Could you check a few things on this model? Use its own coordinates, in mm. A direction names the side the tool comes from. Coordinates: 2 decimals unless noted, no trailing zeros. Order: outer loops, then holes, each group sorted by start corner. A loop starts at its lowest first (then second) coordinate and runs counter-clockwise, first axis right, second up. Notation, with made-up numbers: (47.5, 57.25) - (86.5, 57.25) arc R26 cw to (86.5, 92.25) - close; hole circle Ø4 at (52, 25). An arc over 180 degrees is marked (long way). Answer as CSV lines item,"result". Start each with the question number.
1. I want a section at C-C, the plane z = 0.75. List the corners of the cut face in (x, y) for me, and give its area (3 significant figures).
2. For faces 1 (the face through (0, 2, 2)), 2 (the face through (-5, 0, 2)), which set-ups out of +Z, -Z, +X, -X, +Y, -Y let a thin tool reach every point of the face, with its end or its side?
3. I want a section at B-B, the plane x = 0. List the corners of the cut face in (y, z) for me, and give its area (3 significant figures).
4. I need wall thicknesses on probe 1 along Y at (x, z) = (-2, 0.6); probe 2 along X at (y, z) = (0.9, 1.55). Which ranges of each line are inside material? Lowest first, please.
5. I want a section at A-A, the plane y = -1.55. List the corners of the cut face in (x, z) for me.
6. Thinking about a two-plate mould opening in Y: for faces 3 (the face through (-4, 0, 2)), 4 (the face through (0, 3, 2)), 5 (the face through (0, -3, 2)), which applies, released by +Y, released by -Y, zero draft, split by the parting line, or undercut?
Autodesk Inventor part; units mm, degrees
ref_plane "Work Plane1" through (0, 0, 2) normal (0, 0, 1) x (1, 0, 0)
ref_plane "YZ Plane" through (0, 0, 0) normal (1, 0, 0) x (0, 1, 0)
ref_plane "XZ Plane" through (0, 0, 0) normal (0, 1, 0) x (-1, 0, 0)
sketch "Sketch1" plane through (0, 0, 0) normal (0, 0, 1) x (1, 0, 0)
  line L0 (-4, 2) -> (4, 2)
  line L1 (4, 2) -> (4, -2)
  line L2 (4, -2) -> (-4, -2)
  line L3 (-4, -2) -> (-4, 2)
  line L4 (5, 3) -> (-5, 3)
  line L5 (-5, 3) -> (-5, -3)
  line L6 (-5, -3) -> (5, -3)
  line L7 (5, -3) -> (5, 3)
  point P0 (0, 0)
  dimension "d0" = 8
  dimension "d1" = 4
  dimension "d2" = 2
  dimension "d3" = 4
  dimension "d5" = 1
extrude "Extrusion1" add sketch "Sketch1" along normal blind 4
ref_plane "Work Plane1" through (0, 0, 2) normal (0, 0, 1) x (1, 0, 0)
sketch "Sketch2" plane through (0, 0, 2) normal (0, 0, 1) x (1, 0, 0)
  line L0 (0, 0) -> (5.4411, 0) construction
  point P0 (2.25, 1)
  point P1 (0.75, 1)
  point P2 (-0.75, 1)
  point P3 (-2.25, 1)
  dimension "d11" = 1.5
  dimension "d16" = 2.25
  dimension "d17" = 1
properties part number "CrimpSocket"
Solved:
1,outline,"(-5, -3) - (5, -3) - (5, 3) - (-5, 3) - close; hole (-4, -2) - (4, -2) - (4, 2) - (-4, 2) - close"
1,area,"28.0 mm2"
2,face 1,"+Z, -Z"
2,face 2,"+Z, -Z, -X, +Y, -Y"
3,outline,"(-3, 0) - (-2, 0) - (-2, 4) - (-3, 4) - close; (2, 0) - (3, 0) - (3, 4) - (2, 4) - close"
3,area,"8.00 mm2"
4,probe 1,"y = -3 to -2, 2 to 3"
4,probe 2,"x = -5 to -4, 4 to 5"
5,outline,"(-5, 0) - (-4, 0) - (-4, 4) - (-5, 4) - close; (4, 0) - (5, 0) - (5, 4) - (4, 4) - close"
6,face 3,"undercut"
6,face 4,"released by +Y"
6,face 5,"released by -Y"
